from build123d import *

# Parameters (mm, degrees)
SKETCH1_W                    = 390
SKETCH1_H                    = 90
BOSS_EXTRUDE1_DEPTH          = 3.175
CSK_FOR_M4_SFHCS1_AT_2_COUNT = 2
CSK_FOR_M4_SFHCS1_AT_2_PITCH = 50
CSK_FOR_M4_SFHCS1_AT_3_COUNT = 2
CSK_FOR_M4_SFHCS1_AT_3_PITCH = 30
CSK_FOR_M4_SFHCS1_AT_4_COUNT = 2
CSK_FOR_M4_SFHCS1_AT_4_PITCH = 40
CSK_FOR_M4_SFHCS3_AT_2_COUNT = 2
CSK_FOR_M4_SFHCS3_AT_2_PITCH = 80
SKETCH8_W                    = 80
SKETCH8_H                    = 50
CUT_EXTRUDE1_DEPTH           = 3.175


with BuildPart() as part:
    # Sketch1 → Boss-Extrude1 (new body)
    with BuildSketch(Plane.XY):
        Rectangle(SKETCH1_W, SKETCH1_H)
    extrude(amount=BOSS_EXTRUDE1_DEPTH)

    # Sketch5 → CSK for M4 SFHCS1 (revolve, cut)
    with BuildSketch(Plane(origin=(150, 10, 0), x_dir=(0, 1, 0), z_dir=(1, 0, 0))):
        Polygon((0, 0), (0, 3.175), (2.25, 3.175), (2.25, 2.23), (4.48, 0), align=None)
    csk_for_m4_sfhcs1 = revolve(axis=Axis((150, 10, -6.35), (0, 0, 1)), mode=Mode.SUBTRACT)

    # CSK for M4 SFHCS1 at 2: CSK for M4 SFHCS1 ×2
    with Locations(*[Vector(0.6, -0.8, 0) * (i * CSK_FOR_M4_SFHCS1_AT_2_PITCH) for i in range(1, CSK_FOR_M4_SFHCS1_AT_2_COUNT)]):
        add(csk_for_m4_sfhcs1, mode=Mode.SUBTRACT)

    # CSK for M4 SFHCS1 at 3: CSK for M4 SFHCS1 ×2
    with Locations(*[(i * CSK_FOR_M4_SFHCS1_AT_3_PITCH, 0, 0) for i in range(1, CSK_FOR_M4_SFHCS1_AT_3_COUNT)]):
        add(csk_for_m4_sfhcs1, mode=Mode.SUBTRACT)

    # CSK for M4 SFHCS1 at 4: CSK for M4 SFHCS1 ×2
    with Locations(*[(0, -i * CSK_FOR_M4_SFHCS1_AT_4_PITCH, 0) for i in range(1, CSK_FOR_M4_SFHCS1_AT_4_COUNT)]):
        add(csk_for_m4_sfhcs1, mode=Mode.SUBTRACT)

    # Sketch7 → CSK for M4 SFHCS3 (revolve, cut)
    with BuildSketch(Plane(origin=(190, 40, 3.175), x_dir=(0, -1, 0), z_dir=(1, 0, 0))):
        Polygon((0, 0), (0, 3.175), (2.25, 3.175), (2.25, 2.23), (4.48, 0), align=None)
    csk_for_m4_sfhcs3 = revolve(axis=Axis((190, 40, 9.525), (0, 0, -1)), mode=Mode.SUBTRACT)

    # CSK for M4 SFHCS3 at 2: CSK for M4 SFHCS3 ×2
    with Locations(*[(0, -i * CSK_FOR_M4_SFHCS3_AT_2_PITCH, 0) for i in range(1, CSK_FOR_M4_SFHCS3_AT_2_COUNT)]):
        add(csk_for_m4_sfhcs3, mode=Mode.SUBTRACT)

    # Mirror1: CSK for M4 SFHCS1, CSK for M4 SFHCS3 across plane
    add(csk_for_m4_sfhcs1.mirror(Plane(origin=(0, 0, 0), x_dir=(0, 0, 1), z_dir=(1, 0, 0))), mode=Mode.SUBTRACT)
    add(csk_for_m4_sfhcs3.mirror(Plane(origin=(0, 0, 0), x_dir=(0, 0, 1), z_dir=(1, 0, 0))), mode=Mode.SUBTRACT)

    # Mirror1 copy 1 sketch → Mirror1 copy 1 (revolve, cut)
    with BuildSketch(Plane(origin=(-180, -30, 0), x_dir=(0, 1, 0), z_dir=(-1, 0, 0))):
        Polygon((0, 0), (0, -3.175), (2.25, -3.175), (2.25, -2.23), (4.48, 0), align=None)
    revolve(axis=Axis((-180, -30, -6.35), (0, 0, -1)), mode=Mode.SUBTRACT)

    # Mirror1 copy 2 sketch → Mirror1 copy 2 (revolve, cut)
    with BuildSketch(Plane(origin=(-180, 10, 0), x_dir=(0, 1, 0), z_dir=(-1, 0, 0))):
        Polygon((0, 0), (0, -3.175), (2.25, -3.175), (2.25, -2.23), (4.48, 0), align=None)
    revolve(axis=Axis((-180, 10, -6.35), (0, 0, -1)), mode=Mode.SUBTRACT)

    # Mirror1 copy 3 sketch → Mirror1 copy 3 (revolve, cut)
    with BuildSketch(Plane(origin=(-150, -30, 0), x_dir=(0, 1, 0), z_dir=(-1, 0, 0))):
        Polygon((0, 0), (0, -3.175), (2.25, -3.175), (2.25, -2.23), (4.48, 0), align=None)
    revolve(axis=Axis((-150, -30, -6.35), (0, 0, -1)), mode=Mode.SUBTRACT)

    # Mirror1 copy 4 sketch → Mirror1 copy 4 (revolve, cut)
    with BuildSketch(Plane(origin=(-190, -40, 3.175), x_dir=(0, -1, 0), z_dir=(-1, 0, 0))):
        Polygon((0, 0), (0, -3.175), (2.25, -3.175), (2.25, -2.23), (4.48, 0), align=None)
    revolve(axis=Axis((-190, -40, 9.525), (0, 0, 1)), mode=Mode.SUBTRACT)

    # Sketch8 → Cut-Extrude1 (cut)
    with BuildSketch(Plane.XY.offset(3.175)):
        with Locations((-90, 0)):
            Rectangle(SKETCH8_W, SKETCH8_H)
    extrude(amount=-CUT_EXTRUDE1_DEPTH, mode=Mode.SUBTRACT)


solid = part.part
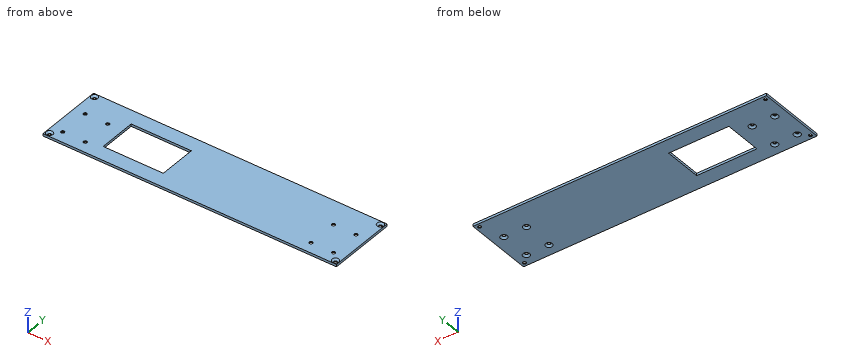
CAD build for the part. Positions are in the model's coordinates, mm. Round coordinates to 2 decimals unless told otherwise and drop trailing zeros. Write each loop counter-clockwise with the first axis right and the second up, starting at its lowest first coordinate (ties: lowest second). Pieces come first, ordered by that corner, then holes.
(1) Slice it at B-B, the plane x = -99. Write the cut outline in (y, z) (3 decimals), and give its area (3 significant figures).
(2) Drop flat-ended pins along their axis: P1, Ø4, axis at x = 180, y = -30, coming from the -Z side; P2, Ø6, axis at x = -190, y = 40, coming from the -Z side; P3, Ø7, axis at x = -150, y = -30, coming from the -Z side; P4, Ø5, axis at x = 190, y = 40, coming from the +Z side (3 decimals). Give the stop position or say it passes through.
(3) Slice it at A-A, the plane y = -15. Write the cut outline in (x, z) (3 decimals).
(4) Slice it at C-C, the plane z = 1.65. Count the separate pieces of the cut face and the enclosed holes in it, and give its area (3 significant figures).
(5) Probe line 1 along Y through (x, z) = (-180, 3); line 2 along X through (y, z) = (-30, 2.9); line 3 along Y through (x, z) = (-190, 0.6). List the from-to ranges inside material, lowest first.
From the geometry:
1. outline: (-45, 0) - (-25, 0) - (-25, 3.175) - (-45, 3.175) - close; (25, 0) - (45, 0) - (45, 3.175) - (25, 3.175) - close
1. area: 127 mm2
2. P1: passes through
2. P2: stops at z = 0
2. P3: stops at z = 0.98
2. P4: stops at z = 1.195
3. outline: (-195, 0) - (-130, 0) - (-130, 3.175) - (-195, 3.175) - close; (-50, 0) - (195, 0) - (195, 3.175) - (-50, 3.175) - close
4. separate pieces: 1
4. enclosed holes: 13
4. area: 30,800 mm2
5. line 1: y = -45 to -32.25, -27.75 to 7.75, 12.25 to 45
5. line 2: x = -195 to -182.25, -177.75 to -152.25, -147.75 to 147.75, 152.25 to 177.75, 182.25 to 195
5. line 3: y = -45 to -42.25, -37.75 to 37.75, 42.25 to 45
